Input: part model. Units: mm. Frame: model coordinates. A direction names the side the tool comes from. Give positions to 0.01 mm unless a question says otherwise; leave off trailing zeros. Write each loop counter-clockwise with the first axis right and the second up, starting at its lowest first coordinate (ties: lowest second). Pieces come first, ordered by that corner, then holes. Notation, with made-up numbers: (72, 21.5) -> (111, 21.5) arc R38 ccw to (111, 60.5) -> close; hole circle Ø11 at (10, 12.25). An arc over 180 degrees is marked (long way). Return JSON: item names as keys, results as strings. Group by question number.
Item 1: Section D-D, the plane y = -118. Count the separate pieces of the cut face and the enclosed holes in it, then the cut area to 3 significant figures.
Item 2: Line query: line 1 (Z direction, x = -39, y = 76); line 2 (Z direction, x = 15.5, y = -109). Output: solid intervals per line, ascending. Write a range as [from, to].
Item 3: Section C-C, the plane z = -2.75. Return loops of the section in (x, y), then the cut area to 3 significant figures.
Item 4: Section B-B, the plane y = 3.5. Return loops of the section in (x, z).
Item 5: Pin query (flat end, axial travel): P1, Ø12, axis at x = -51.5, y = 30, coming from the -Z side. Return the tip coordinate at first contact, or that it passes through.
Item 6: Section A-A, the plane x = -32.5. Return loops of the section in (y, z).
Item 7: Mould query, pull axis X, two halves, no side actions, for faces 1 (the face through (73.5, -130.44, -13.29)), 2 (the face through (-73, 89, 2)), 3 (the face through (48.141, -116.236, -8.168)). Classes: released by +X, released by -X, zero draft, split by the parting line, or undercut.
Item 8: Set-up query: faces 4 (the face through (74, 88, 2)), 5 (the face through (-1, 2, 0)). Return all of +Z, -Z, +X, -X, +Y, -Y with unobstructed straight access to the full face (end or side cutting, diameter ignored); none if empty.
Autodesk Inventor part; units mm, degrees
ref_plane "YZ Plane" through (0, 0, 0) normal (1, 0, 0) x (0, 1, 0)
ref_plane "XZ Plane" through (0, 0, 0) normal (0, 1, 0) x (-1, 0, 0)
ref_plane "XY Plane" through (0, 0, 0) normal (0, 0, 1) x (1, 0, 0)
sketch "Sketch3" plane through (0, 0, 0) normal (0, 0, 1) x (1, 0, 0)
  line L0 (-75, -90) -> (75, -90)
  line L1 (75, -90) -> (75, 90)
  line L2 (75, 90) -> (-75, 90)
  line L3 (-75, 90) -> (-75, -90)
  line L4 (-75, -90) -> (75, 90) construction
  line L5 (75, -90) -> (-75, 90) construction
  point P0 (0, 0)
  dimension "d11" = 150
  dimension "d12" = 180
extrude "Plate3" add sketch "Sketch3" along normal blind 3
sketch "Sketch4" plane through (-75, -88.9739, 0.1809) normal (0, -0.3420201, 0.9396926) x (1, 0, 0)
  line L0 (150, 0) -> (0, 0)
  line L1 (0, 0) -> (0, -45)
  line L2 (0, -45) -> (150, -45)
  line L3 (150, -45) -> (150, 0)
edge flange "Flange2" height 45 angle 20 thickness 3 bend radius 3 thickness toward (0, -0.3420201, 0.9396926) relief tear relief width 3 relief depth 1.5 edges at (0, -90, 0) wall of the first edge with corners at (75, -88.9739, 0.1809) (-75, -88.9739, 0.1809) (-75, -131.2601, -15.21) (75, -131.2601, -15.21)
bend "Bend2"
corner "Corner2"
fillet "Fillet1" radius 5 4 edges at (75, 90, 1.5) (-75, 90, 1.5) (-75, -131.7731, -13.8004) (75, -131.7731, -13.8004)
sketch "Sketch6" plane through (0, 0, 3) normal (0, 0, 1) x (1, 0, 0)
  line L0 (-67.272, 87) -> (67.272, 87) construction
  line L1 (67.272, 87) -> (67.272, -48) construction
  line L2 (67.272, -48) -> (-67.272, -48) construction
  line L3 (-67.272, -48) -> (-67.272, 87) construction
  line L4 (-75, -88.942) -> (75, -88.942)
  line L5 (-70, 90) -> (70, 90)
  point P0 (0, 0)
  point P1 (0, 87)
  point P2 (0, 90)
  dimension "d50" = 178.942
  dimension "d51" = 140
  dimension "d52" = 135
  dimension "d53" = 3
decal "Decal2"
sketch "Sketch7" plane through (-75, -90.9942, 2.6382) normal (0, -0.3420201, 0.9396926) x (1, 0, 0)
  line L0 (150, 0) -> (150, -38.942)
  line L1 (0, -38.942) -> (0, 0)
  line L2 (145, -43.942) -> (5, -43.942)
  point P0 (75, 84.6042)
  point P1 (25, -29.442)
  point P2 (125, -29.442)
  dimension "d62" = 100
  dimension "d63" = 150
  dimension "d64" = 25
  dimension "d65" = 14.5
hole "Hole1" at (-50, -118.6606, -7.4316) at (50, -118.6606, -7.4316) direction (0, 0.3420201, -0.9396926) diameter 5.5 end through all
equation "\"d71\" = Grubosc"
equation "\"d13\" = Grubosc"
equation "\"d14\" = SzerokośćGięciaPodcięcia"
equation "\"d15\" = GłębokośćGięciaPodcięcia"
equation "\"d16\" = MinimalnaPozostałość"
equation "\"d17\" = PromieńPrzejścia"
equation "\"d20\" = PromieńGięcia"
equation "\"d21\" = RozmiarPodcięciaNarożnika"
equation "\"d22\" = Wielk_odstępu"
equation "\"d23\" = Rozmiar_promienia_Jacobiego"
equation "\"PromieńGięcia\" = Grubosc"
equation "\"SzerokośćGięciaPodcięcia\" = Grubosc"
equation "\"GłębokośćGięciaPodcięcia\" = 0.5 * Grubosc"
equation "\"RozmiarPodcięciaNarożnika\" = 4 * Grubosc"
equation "\"MinimalnaPozostałość\" = 2 * Grubosc"
equation "\"PromieńPrzejścia\" = PromieńGięcia"
equation "\"Rozmiar_promienia_Jacobiego\" = PromieńGięcia"
equation "\"Wielk_odstępu\" = Grubosc"
properties part number "fin" material "S235JR(1.0038)"
Answer below:
{
 "1": {"separate pieces": "3", "enclosed holes": "0", "area": "444 mm2"},
 "2": {"line 1": "z = [0, 3]", "line 2": "z = [-7.11, -3.92]"},
 "3": {"outline": "(-75, -105.8) -> (75, -105.8) -> (75, -97.03) -> (-75, -97.03) -> close", "area": "1,320 mm2"},
 "4": {"outline": "(-75, 0) -> (75, 0) -> (75, 3) -> (-75, 3) -> close"},
 "5": {"P1": "stops at z = 0"},
 "6": {"outline": "(-132.29, -12.39) -> (-131.26, -15.21) -> (-89.97, -0.18) arc R3 cw to (-88.94, 0) -> (90, 0) -> (90, 3) -> (-88.94, 3) arc R6 ccw to (-90.99, 2.64) -> close"},
 "7": {"face 1": "released by +X", "face 2": "released by -X", "face 3": "undercut"},
 "8": {"face 4": "+Z, -Z, +X, +Y", "face 5": "-Z, +X, -X, +Y"}
}
